The listing builds one solid part. Answer for the finished solid, in the listing's coordinates (mm). A direction names the side the tool comes from. Give positions to 0.01 mm unless a question says otherwise; leave off trailing zeros. Order: outer loops, then holes, each group sorted by start corner. A loop starts at its lowest first (then second) coordinate and runs counter-clockwise, first axis right, second up. Notation, with made-up numbers: (25, 55) - (76, 55) arc R33 ccw to (76, 91) - close; hole circle Ø6 at (0.25, -35.75). An arc over 180 degrees is marked (long way). Answer in a Markdown table with one row per item. Add a question column.
```python
from build123d import *

# Parameters (mm, degrees)
SALIENTE_EXTRUIR1_DEPTH = 18
CROQUIS4_W              = 23
CROQUIS4_H              = 16
CORTAR_EXTRUIR1_DEPTH   = 1
REDONDEO1_R             = 1


with BuildPart() as part:
    # Croquis2 → Saliente-Extruir1 (new body)
    with BuildSketch(Plane(origin=(0, 0, 0), x_dir=(1, 0, 0), z_dir=(0, 1, 0))):
        Polygon((0, 50), (0, 0), (23, 0), (23, 50), (23, 130), (10.12, 130), (10.12, 50), align=None)
    extrude(amount=SALIENTE_EXTRUIR1_DEPTH)

    # Croquis4 → Cortar-Extruir1 (cut)
    with BuildSketch(Plane.XY):
        with Locations((11.5, 8)):
            Rectangle(CROQUIS4_W, CROQUIS4_H)
    extrude(amount=-CORTAR_EXTRUIR1_DEPTH, mode=Mode.SUBTRACT)

    # Redondeo1
    redondeo1_edges = [part.edges().sort_by_distance(p)[0] for p in [
        (0, 18, -25),
        (11.5, 18, 0),
        (23, 18, -65),
    ]]
    fillet(redondeo1_edges, radius=REDONDEO1_R)


solid = part.part
```
(1) Straight lines are drawn through the part: line 1 (Z direction, x = 13.75, y = 15.75); line 2 (Z direction, x = 5, y = 12.25); line 3 (X direction, y = 2.5, z = -63). For each, find the intervals that lie inside material, in ascending order.
(2) Find section B-B, the plane x = 7.25. Write down the section's boundary in (y, z), plus the area to 3 significant figures.
(3) Each of these flat-tipped pins is pushed along its axis until it touches: P1, Ø10, axis at x = 12, y = 7, coming from the +Z side; P2, Ø2, axis at x = 9, z = -71, coming from the +Y side; P3, Ø8, axis at x = 6, y = 7, coming from the -Z side. Where does it stop, or does it pass through?
(4) Find section A-A, the plane y = 14.5. Write down the section's boundary in (x, z).
(5) For faces 1 (the face through (14, 18, -52)), 2 (the face through (5, 9, -50)), 3 (the face through (11, 8, -1)), determine the directions among +Z, -Z, +X, -X, +Y, -Y from which every point of the face is accessible in a straight line to the end or side of a thin tool.
(6) Find section C-C, the plane z = -80.5. Write down the section's boundary in (x, y), plus the area to 3 significant figures.
Answer key:
| question | item | result |
|---|---|---|
| 1 | line 1 | -130 to -1 |
| 1 | line 2 | -50 to -1 |
| 1 | line 3 | 10.12 to 23 |
| 2 | outline | (0, -50) - (18, -50) - (18, -1) arc R1 ccw to (17, 0) - (16, 0) - (16, -1) - (0, -1) - close |
| 2 | area | 884 mm² |
| 3 | P1 | z = -1 |
| 3 | P2 | through |
| 3 | P3 | z = -50 |
| 4 | outline | (0, -50) - (10.12, -50) - (10.12, -130) - (23, -130) - (23, -1) - (0, -1) - close |
| 5 | face 1 | +Z, -Z, +X, -X, +Y |
| 5 | face 2 | -Z, -X, +Y, -Y |
| 5 | face 3 | +Z, +X, -X, -Y |
| 6 | outline | (10.12, 0) - (23, 0) - (23, 17) arc R1 ccw to (22, 18) - (10.12, 18) - close |
| 6 | area | 232 mm² |
